Study the drawing (mm; zero at the part's minimum x, y, z) and answer. A direction names the side the tool comes from. Coordinates: 2 decimals unless noted, no trailing zeros. Order: outer loops, then holes, each group sorted by start corner. A loop starts at its lowest first (then second) coordinate and runs counter-clockwise, first axis right, second up. Notation, with made-up numbers: (72.25, 4.25) -> (98.25, 4.25) arc R29 cw to (98.25, 34.25) -> close; hole circle Ø5 at (-33, 59.5). An arc over 180 degrees is marked (long way). Answer as CSV lines item,"result". Start each with the question number.
Item 1: Straight lines are drawn through the part: L1, parallel to X at y = 4, z = 38.5; L2, parallel to X at y = 5.25, z = 9.5; L3, parallel to X at y = 8.5, z = 41. For each, find the intervals that lie inside material, in ascending order.
Item 2: Which of the six approach directions +Z, -Z, +X, -X, +Y, -Y give full straight-line access (tool end or side, diameter ignored) to the marked faces 5, 6 and 7?
Item 3: Section A-A (x = 5) is taken. Write down the section's boundary in (y, z).
Item 4: For a pull along X with two mould halves and no side action, classify the marked faces 1, 2, 3 and 4 as pulls with the +X half, pulls with the -X half, needs draft (parallel to the pull), parting line crosses it, or undercut.
Item 5: Section B-B (z = 17.5) is taken. Write down the section's boundary in (x, y), then the cut area to 3 significant figures.
Item 6: Each of these flat-tipped pins is pushed along its axis until it touches: pin 1 Ø3 at (x, y) = (30, 7.5) entering from +Z; pin 2 Ø1.5 at (x, z) = (21.995, 14.825) entering from +Y. Where does it stop, or does it pass through?
Item 7: Section C-C (z = 39) is taken. Write down the section's boundary in (x, y), then the cut area to 3 significant figures.
Item 8: Section D-D (y = 3.25) is taken. Write down the section's boundary in (x, z) (3 decimals), then the cut area to 3 significant figures.
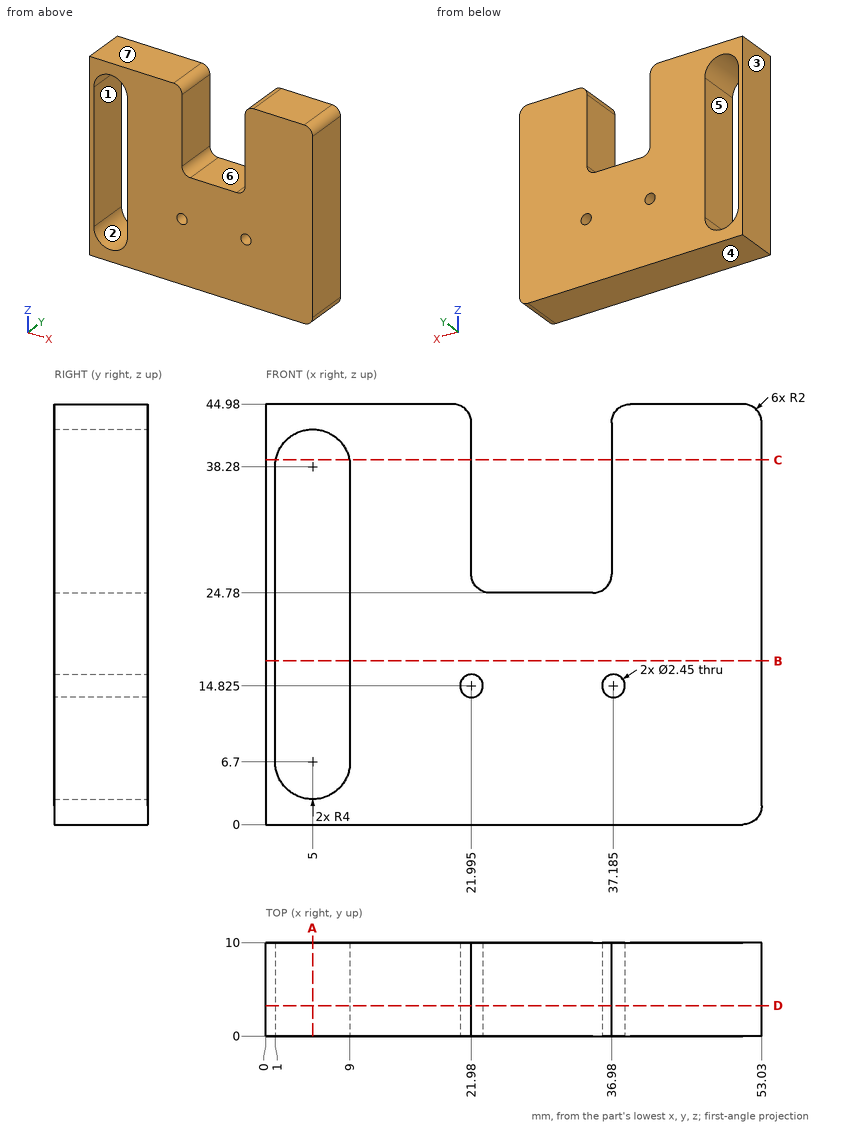
Checked values:
1,L1,"x = 0 to 1.01, 8.99 to 21.98, 36.98 to 53.03"
1,L2,"x = 0 to 1, 9 to 53.03"
1,L3,"x = 0 to 2.07, 7.93 to 21.98, 36.98 to 53.03"
2,face 5,"+Y, -Y"
2,face 6,"+Z, +Y, -Y"
2,face 7,"+Z, +X, -X, +Y, -Y"
3,outline,"(0, 0) -> (10, 0) -> (10, 2.7) -> (0, 2.7) -> close; (0, 42.28) -> (10, 42.28) -> (10, 44.98) -> (0, 44.98) -> close"
4,face 1,"undercut"
4,face 2,"undercut"
4,face 3,"pulls with the -X half"
4,face 4,"needs draft"
5,outline,"(0, 0) -> (1, 0) -> (1, 10) -> (0, 10) -> close; (9, 0) -> (53.03, 0) -> (53.03, 10) -> (9, 10) -> close"
5,area,"450 mm^2"
6,pin 1,"stops at z = 24.78"
6,pin 2,"passes through"
7,outline,"(0, 0) -> (1.07, 0) -> (1.07, 10) -> (0, 10) -> close; (8.93, 0) -> (21.98, 0) -> (21.98, 10) -> (8.93, 10) -> close; (36.98, 0) -> (53.03, 0) -> (53.03, 10) -> (36.98, 10) -> close"
7,area,"302 mm^2"
8,outline,"(0, 0) -> (51.03, 0) arc R2 ccw to (53.03, 2) -> (53.03, 42.98) arc R2 ccw to (51.03, 44.98) -> (38.98, 44.98) arc R2 ccw to (36.98, 42.98) -> (36.98, 26.78) arc R2 cw to (34.98, 24.78) -> (23.98, 24.78) arc R2 cw to (21.98, 26.78) -> (21.98, 42.98) arc R2 ccw to (19.98, 44.98) -> (0, 44.98) -> close; hole (1, 6.7) arc R4 ccw to (9, 6.7) -> (9, 38.28) arc R4 ccw to (1, 38.28) -> close; hole circle Ø2.45 at (21.995, 14.825); hole circle Ø2.45 at (37.185, 14.825)"
8,area,"1,770 mm^2"
